For this review, use the dimensioned drawing (mm, ordinates from the lowest corner) and the shaded views. Coordinates: 2 decimals unless noted, no trailing zeros. Write each loop counter-clockwise with the first axis right and the second up, starting at its lowest first coordinate (ties: lowest second). Pieces come first, ordered by that corner, then holes. Notation, with made-up numbers: M 51.5,66 L 82.5,66 A24 ccw 82.5,103 Z; hole C -5.75,89 d8. An arc over 180 degrees is marked long. One line per question, with ' | ' between items.
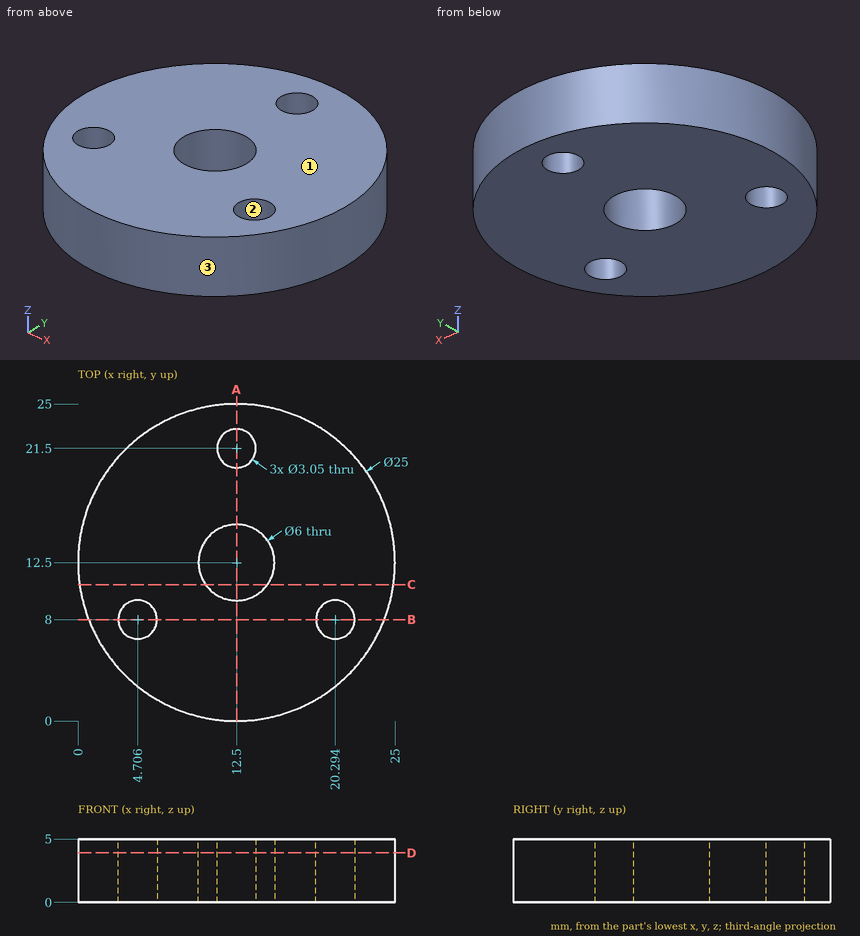
1) We need section C-C on y = 10.75. State the section outline as (x, z) points, then the cut area to 3 significant figures.
Responses:
outline: M 0.12,0 L 10.06,0 L 10.06,5 L 0.12,5 Z; M 14.94,0 L 24.88,0 L 24.88,5 L 14.94,5 Z | area: 99.4 mm^2
2) To check wall thickness, follow line 1 along Y through (x, z) = (12.5, 1.2) (3 decimals); line 2 along X through (y, z) = (8.5, 2.5) (1 decimal); line 3 along X through (y, z) = (10.75, 0.35). State the ranges of each line that lie inside material, in increasing order. Write a range as [from, to].
Responses:
line 1: [0, 9.5], [15.5, 19.975], [23.025, 25] | line 2: [0.7, 3.3], [6.1, 18.9], [21.7, 24.3] | line 3: [0.12, 10.06], [14.94, 24.88]
3) We need section B-B on y = 8. State the section outline as (x, z) points, then the cut area to 3 significant figures.
Responses:
outline: M 0.84,0 L 3.18,0 L 3.18,5 L 0.84,5 Z; M 6.23,0 L 18.77,0 L 18.77,5 L 6.23,5 Z; M 21.82,0 L 24.16,0 L 24.16,5 L 21.82,5 Z | area: 86.1 mm^2
4) Insertion check: pin 1 Ø3 at (y, z) = (9, 4.5) entering from +X; pin 2 Ø3 at (x, z) = (21.5, 2) entering from -Y. Each pin has a flat end and moves straight along its axis. Give the tip position at first contact, or say it passes through.
Responses:
pin 1: x = 24.84 | pin 2: y = 2.5
5) We need section A-A on x = 12.5. State the section outline as (y, z) points (3 decimals).
Responses:
outline: M 0,0 L 9.5,0 L 9.5,5 L 0,5 Z; M 15.5,0 L 19.975,0 L 19.975,5 L 15.5,5 Z; M 23.025,0 L 25,0 L 25,5 L 23.025,5 Z
6) We need section D-D on z = 3.9. State how many separate pieces and enclosed holes the cut face has, then the cut area to 3 significant figures.
Responses:
separate pieces: 1 | enclosed holes: 4 | area: 441 mm^2
7) The part is to be moulded in two halves that separate along Y. For the marked faces 1, 2 and 3, say which applies: +Y half, -Y half, draft (parallel to the pull), parting line (faces both ways), or undercut.
Responses:
face 1: draft | face 2: undercut | face 3: parting line
